Geometry: final body of the model. Coordinates: model frame, mm. Face numbers are marked on the shaded views. A direction names the side the tool comes from. Coordinates: 2 decimals unless noted, no trailing zeros. Loops run counter-clockwise (first coordinate to the right, second up) from the corner with the lowest first, then second, coordinate; pieces in that order, holes last. Notation, with made-up numbers: (76.25, 45.25) - (134.25, 45.25) arc R15 cw to (134.25, 65.25) - close; hole circle Ø4 at (85.25, 17). An arc over 180 degrees is marked (long way). Answer in a Markdown table with one row per item.
Autodesk Inventor part; units mm, degrees
ref_plane "YZ Plane" through (0, 0, 0) normal (1, 0, 0) x (0, 1, 0)
ref_plane "XZ Plane" through (0, 0, 0) normal (0, 1, 0) x (-1, 0, 0)
ref_plane "XY Plane" through (0, 0, 0) normal (0, 0, 1) x (1, 0, 0)
sketch "Esquisse1" plane through (0, 0, 0) normal (0, 1, 0) x (-1, 0, 0)
  circle A0 centre (0, 0) radius 13
  dimension "d0" = 26
extrude "Extrusion1" add sketch "Esquisse1" along normal blind 1
sketch "Esquisse2" plane through (0, 1, 0) normal (0, 1, 0) x (1, 0, 0)
  circle A0 centre (0, 0) radius 13
  circle A1 centre (0, 0) radius 11.675
  dimension "d3" = 23.35
extrude "Extrusion2" add sketch "Esquisse2" along normal blind 8 contours A1
sketch "Esquisse3" plane through (0, 9, 0) normal (0, 1, 0) x (1, 0, 0)
  circle A0 centre (0, 0) radius 11.675
  circle A1 centre (0, 0) radius 13
  dimension "d6" = 26
extrude "Extrusion3" add sketch "Esquisse3" along normal blind 1 contours A0 | A1
sketch "Esquisse4" plane through (0, 10, 0) normal (0, 1, 0) x (1, 0, 0)
  circle A0 centre (0, 0) radius 13
  circle A1 centre (0, 0) radius 8
  dimension "d9" = 16
extrude "Extrusion4" add sketch "Esquisse4" along normal blind 6 contours A1
sketch "Esquisse5" plane through (0, 16, 0) normal (0, 1, 0) x (1, 0, 0)
  circle A0 centre (0, 0) radius 8
  circle A1 centre (0, 0) radius 3
  dimension "d12" = 6
extrude "Extrusion5" cut sketch "Esquisse5" against normal through all contours A1
properties part number "poulie_conrad_209515"
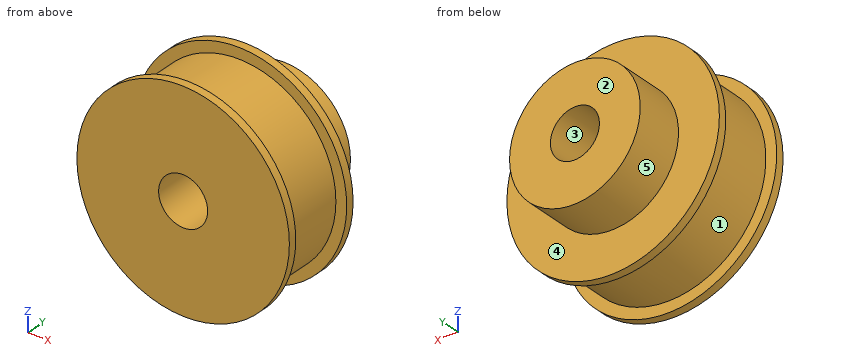
(1) Cut plane D-D on x = -5.5. Output: boundary loops of the cut face in (y, z).
Verdict:
| item | result |
|---|---|
| outline | (0, -11.78) - (1, -11.78) - (1, -10.3) - (9, -10.3) - (9, -11.78) - (10, -11.78) - (10, -5.81) - (16, -5.81) - (16, 5.81) - (10, 5.81) - (10, 11.78) - (9, 11.78) - (9, 10.3) - (1, 10.3) - (1, 11.78) - (0, 11.78) - close |
(2) First-contact query: pin 1 Ø6 at (y, z) = (4, 9.5) entering from -X; pin 2 Ø4 at (y, z) = (10.5, 3.5) entering from -X; pin 3 Ø1 at (y, z) = (9, 5) entering from -X. Flat tips, straight axial feed; report the tip coordinate or a pass-through.
Verdict:
| item | result |
|---|---|
| pin 1 | stops at x = -9.7 |
| pin 2 | stops at x = -12.91 |
| pin 3 | stops at x = -12.2 |
(3) Cut plane A-A on z = 0. Output: boundary loops of the cut face in (x, y) (3 decimals), then the cut area to 3 significant figures.
Verdict:
| item | result |
|---|---|
| outline | (-13, 0) - (-3, 0) - (-3, 16) - (-8, 16) - (-8, 10) - (-13, 10) - (-13, 9) - (-11.675, 9) - (-11.675, 1) - (-13, 1) - close; (3, 0) - (13, 0) - (13, 1) - (11.675, 1) - (11.675, 9) - (13, 9) - (13, 10) - (8, 10) - (8, 16) - (3, 16) - close |
| area | 239 mm² |
(4) Ray query, probe 1 along Z at (x, y) = (0, 12.75); probe 2 along Z at (x, y) = (0, 8) (3 decimals); probe 3 along Y at (x, z) = (-8.5, -8.25). Return the intervals inside material, ascending.
Verdict:
| item | result |
|---|---|
| probe 1 | z = -8 to -3, 3 to 8 |
| probe 2 | z = -11.675 to -3, 3 to 11.675 |
| probe 3 | y = 0 to 1, 9 to 10 |
(5) Cut plane B-B on x = 0. Output: boundary loops of the cut face in (y, z) (3 decimals).
Verdict:
| item | result |
|---|---|
| outline | (0, -13) - (1, -13) - (1, -11.675) - (9, -11.675) - (9, -13) - (10, -13) - (10, -8) - (16, -8) - (16, -3) - (0, -3) - close; (0, 3) - (16, 3) - (16, 8) - (10, 8) - (10, 13) - (9, 13) - (9, 11.675) - (1, 11.675) - (1, 13) - (0, 13) - close |
(6) Cut plane C-C on y = 13. Output: boundary loops of the cut face in (x, z), then the cut area to 3 significant figures.
Verdict:
| item | result |
|---|---|
| outline | circle Ø16 at (0, 0); hole circle Ø6 at (0, 0) |
| area | 173 mm² |
(7) Access query for the marked faces 1 and 2. Directions: +Z, -Z, +X, -X, +Y, -Y. A direction counts if a zero-diameter tool reaches every point of the face in a straight line with its end or side. Return the directions, or none.
Verdict:
| item | result |
|---|---|
| face 1 | none |
| face 2 | +Z, -Z, +X, -X, +Y |
(8) Pull-direction query (Z, two-part tool) for the marked faces 3, 4 and 5; classes: pulls with the +Z half, pulls with the -Z half, needs draft (parallel to the pull), parting line crosses it, or undercut.
Verdict:
| item | result |
|---|---|
| face 3 | undercut |
| face 4 | needs draft |
| face 5 | parting line crosses it |
